Verification items for this drawing (mm, ordinates from the low corner). Round coordinates to 2 decimals unless told otherwise and drop trailing zeros. Order: outer loops, then holes, each group sorted by start corner. A loop starts at its lowest first (then second) coordinate and runs counter-clockwise, first axis right, second up. Notation, with made-up numbers: M 13.25,77.5 L 39.25,77.5 A25 cw 39.25,95.5 Z; hole C 65.25,59.25 d4. An arc over 180 degrees is marked long. Return JSON: item names as keys, results as strings. Group by question number.
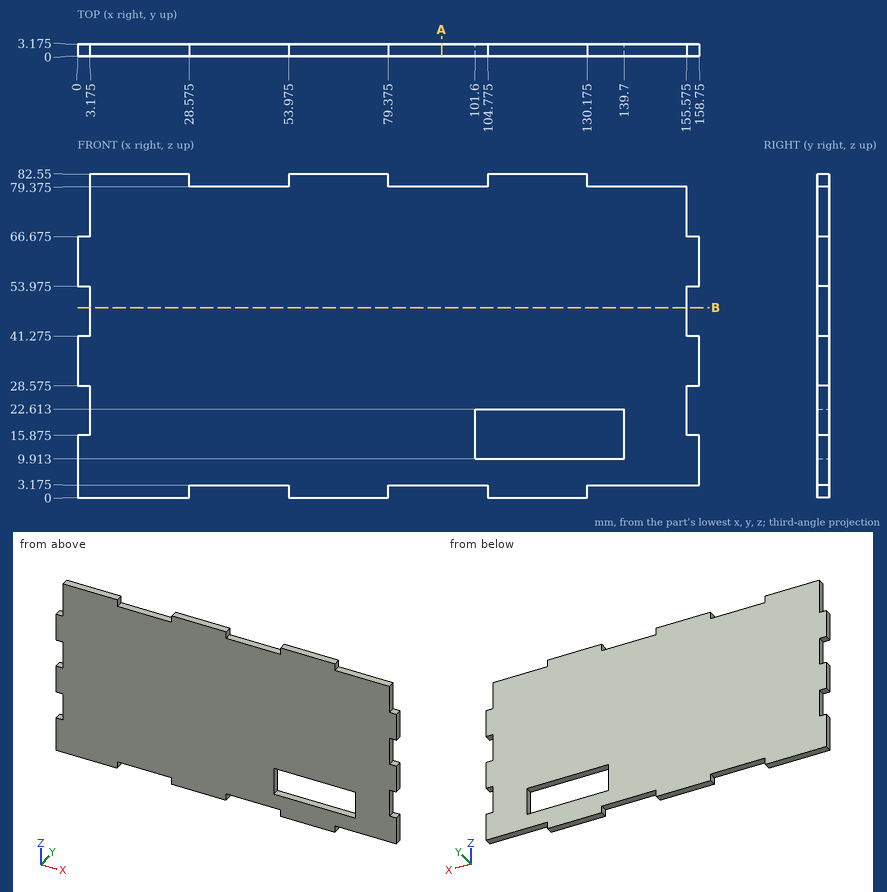
1. Go/stop test with flat-tipped pins: pin 1 (1 mm diameter, centred on y = 1, z = 50.5, fed in from -X) (3 decimals); pin 2 (1 mm diameter, centred on x = 143.5, y = 1.5, fed in from +Z) (3 decimals). Record where each tip stops, or that it passes through.
2. Thickness scan on line 1 along X through (y, z) = (0.3, 21) (3 decimals); line 2 along X through (y, z) = (2.9, 68) (3 decimals); line 3 along Z through (x, y) = (34, 1.1) (3 decimals). Record the ranges inside material, lowest first. Write a range as from..to.
3. Cross-section at B-B (z = 48.5). Enter the section's corners in (x, y) (3 decimals).
4. Cross-section at A-A (x = 93). Enter the section's corners in (y, z) (3 decimals), plus the area to 3 significant figures.
Computed:
{
 "1": {"pin 1": "stops at x = 3.175", "pin 2": "stops at z = 79.375"},
 "2": {"line 1": "x = 3.175..101.6, 139.7..155.575", "line 2": "x = 3.175..155.575", "line 3": "z = 3.175..79.375"},
 "3": {"outline": "M 3.175,0 L 155.575,0 L 155.575,3.175 L 3.175,3.175 Z"},
 "4": {"outline": "M 0,3.175 L 3.175,3.175 L 3.175,79.375 L 0,79.375 Z", "area": "242 mm²"}
}
